The listing builds one solid part. Answer for the finished solid, in the listing's coordinates (mm). A direction names the side the tool comes from. Coordinates: 2 decimals unless noted, no trailing zeros. Write each loop counter-clockwise with the first axis right and the second up, starting at its lowest first coordinate (ties: lowest second). Pieces come first, ordered by that corner, then holes. Notation, with made-up numbers: M 72,56 L 84,56 A22 cw 84,89 Z; hole C 86,-35 d3. An arc over 180 degrees is marked long. Answer as CSV lines item,"result".
```python
from build123d import *

# Parameters (mm, degrees)
F0_R     = 2.1
F1_DEPTH = 170


with BuildPart() as f1:
    # F0 (on Front) → F1 (new body)
    with BuildSketch(Plane.XZ):
        with BuildLine():
            Line((4.585786, 6), (0, 6))
            Line((0, 6), (-4.585786, 6))
            Line((-4.585786, 6), (-8.25, 9.664214))
            Line((-8.25, 9.664214), (-8.25, 13))
            Line((-8.25, 13), (-4, 13))
            Line((-4, 13), (-4, 15))
            Line((-4, 15), (-13, 15))
            ThreePointArc((-13, 15), (-14.414214, 14.414214), (-15, 13))
            Line((-15, 13), (-15, 4))
            Line((-15, 4), (-13, 4))
            Line((-13, 4), (-13, 8.25))
            Line((-13, 8.25), (-9.664214, 8.25))
            Line((-9.664214, 8.25), (-6, 4.585786))
            Line((-6, 4.585786), (-6, 0))
            Line((-6, 0), (-6, -4.585786))
            Line((-6, -4.585786), (-9.664214, -8.25))
            Line((-9.664214, -8.25), (-13, -8.25))
            Line((-13, -8.25), (-13, -4))
            Line((-13, -4), (-15, -4))
            Line((-15, -4), (-15, -13))
            ThreePointArc((-15, -13), (-14.414214, -14.414214), (-13, -15))
            Line((-13, -15), (-4, -15))
            Line((-4, -15), (-4, -13))
            Line((-4, -13), (-8.25, -13))
            Line((-8.25, -13), (-8.25, -9.664214))
            Line((-8.25, -9.664214), (-4.585786, -6))
            Line((-4.585786, -6), (0, -6))
            Line((0, -6), (4.585786, -6))
            Line((4.585786, -6), (8.25, -9.664214))
            Line((8.25, -9.664214), (8.25, -13))
            Line((8.25, -13), (4, -13))
            Line((4, -13), (4, -15))
            Line((4, -15), (13, -15))
            ThreePointArc((13, -15), (14.414214, -14.414214), (15, -13))
            Line((15, -13), (15, -4))
            Line((15, -4), (13, -4))
            Line((13, -4), (13, -8.25))
            Line((13, -8.25), (9.664214, -8.25))
            Line((9.664214, -8.25), (6, -4.585786))
            Line((6, -4.585786), (6, 0))
            Line((6, 0), (6, 4.585786))
            Line((6, 4.585786), (9.664214, 8.25))
            Line((9.664214, 8.25), (13, 8.25))
            Line((13, 8.25), (13, 4))
            Line((13, 4), (15, 4))
            Line((15, 4), (15, 13))
            ThreePointArc((15, 13), (14.414214, 14.414214), (13, 15))
            Line((13, 15), (4, 15))
            Line((4, 15), (4, 13))
            Line((4, 13), (8.25, 13))
            Line((8.25, 13), (8.25, 9.664214))
            Line((8.25, 9.664214), (4.585786, 6))
        make_face()
        with Locations((-11.6, -11.6)):
            Circle(F0_R, mode=Mode.SUBTRACT)
        with Locations((11.6, -11.6)):
            Circle(F0_R, mode=Mode.SUBTRACT)
        with Locations((-11.6, 11.6)):
            Circle(F0_R, mode=Mode.SUBTRACT)
        with BuildLine():
            ThreePointArc((-3.4, 0), (-2.404163, 2.404163), (0, 3.4))
            ThreePointArc((0, 3.4), (2.404163, 2.404163), (3.4, 0))
            ThreePointArc((3.4, 0), (2.404163, -2.404163), (0, -3.4))
            ThreePointArc((0, -3.4), (-2.404163, -2.404163), (-3.4, 0))
        make_face(mode=Mode.SUBTRACT)
        with Locations((11.6, 11.6)):
            Circle(F0_R, mode=Mode.SUBTRACT)
    extrude(amount=F1_DEPTH)


solid = f1.part
```
Q1. Straight lines are drawn through the part: line 1 (Z direction, x = -11.6, y = -56); line 2 (Z direction, x = -8, y = -70); line 3 (X direction, y = -15, z = 11). For each, find the intervals that lie inside material, in ascending order.
Output:
line 1,"-15 to -13.7, -9.5 to -8.25, 8.25 to 9.5, 13.7 to 15"
line 2,"-15 to -13, -9.41 to -6.59, 6.59 to 9.41, 13 to 15"
line 3,"-15 to -13.61, -9.59 to -8.25, 8.25 to 9.59, 13.61 to 15"
Q2. The mould has two halves that part along X. Classify faces 1 (the flat face through (-4, -170, 0)), 2 (the flat face through (15, -84, 8)), 3 (the flat face through (7.858, -83.81, -6.444)): pulls with the +X half, pulls with the -X half, needs draft (parallel to the pull), parting line crosses it, or undercut.
Output:
face 1,"needs draft"
face 2,"pulls with the +X half"
face 3,"undercut"
Q3. Find section A-A (z = 1.5). Give the vertices of the cut face in (x, y).
Output:
outline,"M -6,-170 L -3.05,-170 L -3.05,0 L -6,0 Z; M 3.05,-170 L 6,-170 L 6,0 L 3.05,0 Z"
Q4. For faces 4 (the flat face through (-6, -84, 0)), 5 (the flat face through (-15, -84, -8)), determine the directions among +Z, -Z, +X, -X, +Y, -Y from which every point of the face is accessible in a straight line to the end or side of a thin tool.
Output:
face 4,"+Y, -Y"
face 5,"+Z, -Z, -X, +Y, -Y"
Q5. Flat-ended cylindrical pins translate along their axes: pin 1 Ø2 at (x, y) = (0, -140) entering from +Z; pin 2 Ø10 at (x, z) = (-1, -1) entering from +Y; pin 3 Ø1 at (y, z) = (-90.5, 1) entering from -X; pin 4 Ø1 at (x, y) = (14.5, -116.5) entering from +Z. Find the tip coordinate at first contact, or state that the pin passes through.
Output:
pin 1,"z = 6"
pin 2,"y = 0"
pin 3,"x = -6"
pin 4,"z = 14.73"
Q6. Find section B-B (y = -49). Count the separate pieces of the cut face and the enclosed holes in it, and give its area (3 significant figures).
Output:
separate pieces,"1"
enclosed holes,"5"
area,"333 mm2"
